Autodesk Inventor part; units mm, degrees
ref_plane "YZ Plane" through (0, 0, 0) normal (1, 0, 0) x (0, 1, 0)
ref_plane "XZ Plane" through (0, 0, 0) normal (0, 1, 0) x (-1, 0, 0)
ref_plane "XY Plane" through (0, 0, 0) normal (0, 0, 1) x (1, 0, 0)
sketch "Sketch1" plane through (0, 0, 0) normal (0, 1, 0) x (-1, 0, 0)
  line L0 (11, -4.5) -> (-11, -4.5)
  line L1 (-11, -4.5) -> (-11, 4.5)
  line L2 (-11, 4.5) -> (11, 4.5)
  line L3 (11, 4.5) -> (11, -4.5)
  line L4 (11, -4.5) -> (-11, 4.5) construction
  line L5 (-11, -4.5) -> (11, 4.5) construction
  point P0 (0, 0)
  dimension "d0" = 22
  dimension "d1" = 9
extrude "Extrusion1" add sketch "Sketch1" along normal mid plane 3
sketch "Sketch2" plane through (-11, 1.5, 4.5) normal (0, 0, 1) x (1, 0, 0)
  line L0 (11, 9) -> (11, 9)
  line L1 (16.5, 3.5) -> (16.5, 0)
  line L2 (16.5, 0) -> (5.5, 0)
  line L3 (5.5, 0) -> (5.5, 3.5)
  line L4 (22, 0) -> (0, 0)
  line L5 (5.5, 4.5) -> (16.5, -4.5) construction
  line L6 (16.5, 4.5) -> (5.5, -4.5) construction
  arc A0 (11, 9) -> (5.5, 3.5) centre (11, 3.5) ccw
  arc A1 (16.5, 3.5) -> (11, 9) centre (11, 3.5) ccw
  point P0 (11, -1.5)
  point P1 (16.5, 9)
  point P2 (11, 0)
  dimension "d4" = 11
  dimension "d5" = 9
  dimension "d6" = 0
  dimension "d7" = 5.5
extrude "Extrusion2" add sketch "Sketch2" against normal blind 9
sketch "Sketch3" plane through (-11, -1.5, 4.5) normal (0, 0, 1) x (1, 0, 0)
  circle A0 centre (11, 6.5) radius 5
  line L0 (5.5, 6.5) -> (5.5, 3)
  point P0 (11, 1.5)
  dimension "d10" = 10
  dimension "d11" = 5.5
extrude "Extrusion3" add sketch "Sketch3" along normal blind 1.5
sketch "Sketch4" plane through (11, -1.5, -4.5) normal (0, 0, -1) x (-1, 0, 0)
  arc A0 (16.5, 6.5) -> (5.5, 6.5) centre (11, 6.5) ccw
  circle A1 centre (11, 6.5) radius 5
  point P0 (11, 1.5)
  dimension "d14" = 10
extrude "Extrusion4" add sketch "Sketch4" along normal blind 3
sketch "Sketch5" plane through (0, 5, -7.5) normal (0, 0, -1) x (-1, 0, 0)
  circle A0 centre (0, 0) radius 3.5
  point P0 (0, -5)
  dimension "d17" = 7
extrude "Extrusion5" cut sketch "Sketch5" against normal through all
sketch "Sketch6" plane through (0, -1.5, 0) normal (0, -1, 0) x (1, 0, 0)
  circle A0 centre (-8, 0) radius 1.5
  line L0 (-11, 4.5) -> (-11, -4.5)
  point P0 (0, 0)
  dimension "d20" = 3
  dimension "d21" = 3
extrude "Extrusion6" cut sketch "Sketch6" against normal through all
sketch "Sketch7" plane through (0, -1.5, 0) normal (0, -1, 0) x (1, 0, 0)
  circle A0 centre (8, 0) radius 1.5
  line L0 (11, -4.5) -> (11, 4.5)
  point P0 (0, 0)
  dimension "d24" = 3
  dimension "d25" = 3
extrude "Extrusion7" cut sketch "Sketch7" against normal through all
sketch "Sketch8" plane through (0, -1.5, 0) normal (0, -1, 0) x (1, 0, 0)
  circle A0 centre (0, 0) radius 1.5
  dimension "d28" = 3
hole "Hole1" at (0, -1.5, 0) direction (0, 1, 0) diameter 1 depth 3.04 tip angle 118 countersink diameter 3 countersink angle 90
properties material "Brass, Soft Yellow, Welded"
Read the model definition and answer for the solid it produces. Units are mm, in the model's axes. A direction names the side the tool comes from. Coordinates: 2 decimals unless noted, no trailing zeros. Loops run counter-clockwise (first coordinate to the right, second up) from the corner with the lowest first, then second, coordinate; pieces in that order, holes last.
(1) Consider line 1 along Z through (x, y) = (0, 1.15); line 2 along Z through (x, y) = (-8, -0.3); line 3 along Y through (x, z) = (7.5, 3.25). Determine where each line is inside the solid, lowest interval first.
Solution:
line 1: z = -7.5 to -0.5, 0.5 to 6
line 2: z = -4.5 to -1.5, 1.5 to 4.5
line 3: y = -1.5 to 1.5
(2) A tool of negligible diameter and unlimited length cuts with its end or side. For faces 5 (the face through (-4, 8, 5)), 6 (the face through (5.5, 3, 0)), 7 (the face through (-0.1, -0.4, -4.5)), 8 (the face through (-9.4, 1.5, 1.1)), from which of +Z, -Z, +X, -X, +Y, -Y can it reach the whole face along a straight path? Write none if from no direction.
Solution:
face 5: +Z
face 6: +Z, -Z, +X, +Y
face 7: -Z
face 8: +Z, -Z, -X, +Y
(3) The part is cut by section D-D (z = -5). Determine the outline of the cut face in (x, y).
Solution:
outline: circle Ø10 at (0, 5); hole circle Ø7 at (0, 5)
(4) The part is cut by section A-A (z = 0). Determine the outline of the cut face in (x, y).
Solution:
outline: (-11, -1.5) - (-9.5, -1.5) - (-9.5, 1.5) - (-11, 1.5) - close; (-6.5, -1.5) - (-1.5, -1.5) - (-0.5, -0.5) - (-0.5, 1.54) arc R3.5 cw (long way) to (0.5, 1.54) - (0.5, -0.5) - (1.5, -1.5) - (6.5, -1.5) - (6.5, 1.5) - (5.5, 1.5) - (5.5, 5) arc R5.5 ccw to (-5.5, 5) - (-5.5, 1.5) - (-6.5, 1.5) - close; (9.5, -1.5) - (11, -1.5) - (11, 1.5) - (9.5, 1.5) - close
(5) The part is cut by section B-B (x = 0). Determine the outline of the cut face in (y, z).
Solution:
outline: (-1.5, -4.5) - (0, -4.5) - (0, -7.5) - (1.5, -7.5) - (1.5, -0.5) - (-0.5, -0.5) - (-1.5, -1.5) - close; (-1.5, 1.5) - (-0.5, 0.5) - (1.5, 0.5) - (1.5, 6) - (0, 6) - (0, 4.5) - (-1.5, 4.5) - close; (8.5, -7.5) - (10, -7.5) - (10, -4.5) - (10.5, -4.5) - (10.5, 4.5) - (10, 4.5) - (10, 6) - (8.5, 6) - close
(6) Flat-ended cylindrical pins translate along their axes: pin 1 Ø1.5 at (x, y) = (5, 1) entering from -Z; pin 2 Ø6.5 at (x, y) = (0, 5) entering from +Z; pin 3 Ø3 at (x, z) = (7.5, 0) entering from +Y; pin 4 Ø1.8 at (y, z) = (2.5, 1.5) entering from +X. Find the tip coordinate at first contact, or state that the pin passes through.
Solution:
pin 1: stops at z = -4.5
pin 2: passes through
pin 3: stops at y = 1.5
pin 4: stops at x = 5.5
(7) The mould has two halves that part along X. Classify faces 1 (the face through (-9.5, -0.02, 0.07)), 2 (the face through (0, -1.5, 2)), 3 (the face through (6.5, -0.02, 0.07)), 4 (the face through (-11, 0, 0)): released by +X, released by -X, zero draft, split by the parting line, or undercut.
Solution:
face 1: undercut
face 2: zero draft
face 3: undercut
face 4: released by -X
(8) The part is cut by section C-C (x = -8). Determine the outline of the cut face in (y, z), and give its area (3 significant figures).
Solution:
outline: (-1.5, -4.5) - (1.5, -4.5) - (1.5, -1.5) - (-1.5, -1.5) - close; (-1.5, 1.5) - (1.5, 1.5) - (1.5, 4.5) - (-1.5, 4.5) - close
area: 18.0 mm2
